Build history of the part. All positions in model axes, mm. Coordinates: 2 decimals unless noted, no trailing zeros. Loops run counter-clockwise (first coordinate to the right, second up) from the corner with the lowest first, then second, coordinate; pieces in that order, holes last.
Item 1: Cut at A-A (x = 17). List the corners of the cut face in (y, z), and give its area (3 significant figures).
Item 2: Mould opens along Y. For faces 1 (the face through (61.625, 0.33, 7.493)), 2 (the face through (111.122, -0.205, -0.427)), 3 (the face through (0, 0, 0)), 4 (the face through (123.36, -0.21, 0.18)) say: released by +Y, released by -Y, zero draft, split by the parting line, or undercut.
Item 3: Drill centre lines: line 1 along X through (y, z) = (-0.75, 0.25); line 2 along X through (y, z) = (-0.75, -0.5); line 3 along Z through (x, y) = (90, -0.25). Where is each one in solid material? Low to high.
Item 4: Flat gauge pins, fed straight in: pin 1 (6 mm diameter, centred on x = 62.5, z = -5, fed in from -Y); pin 2 (5 mm diameter, centred on x = 12.5, z = -4, fed in from +Y); pin 3 (8 mm diameter, centred on x = 43.5, y = 4, fed in from +Z); pin 4 (6 mm diameter, centred on x = 108.5, z = -4, fed in from +Y). Where does each tip first touch, or does it go through?
from build123d import *

# Parameters (mm, degrees)
SKETCH1_R                       = 7.5
BOSS_EXTRUDE1_DEPTH             = 125
F_3_32_0_09375_DIAMETER_HOLE1_D = 2.38125
F_2MM_DIAMETER_HOLE_D           = 2


with BuildPart() as part:
    # Sketch1 → Boss-Extrude1 (new body)
    with BuildSketch(Plane(origin=(0, 0, 0), x_dir=(0, 0, -1), z_dir=(1, 0, 0))):
        Circle(SKETCH1_R)
    extrude(amount=BOSS_EXTRUDE1_DEPTH)

    # 3/32 (0.09375) Diameter Hole1 (through all)
    with Locations(Plane(origin=(122.197095896, -2.4168895, -7.099904587), x_dir=(0, -0.946653944928, 0.322251933358), z_dir=(0, -0.322251933358, -0.946653944928))):
        with Locations((0, 0)):
            Hole(F_3_32_0_09375_DIAMETER_HOLE1_D / 2)

    # 2mm Diameter Hole (through all)
    with Locations(Plane(origin=(112.009618943, 7.312828958, -1.665092378), x_dir=(0, 0.222012317051, 0.975043861105), z_dir=(0, 0.975043861105, -0.222012317051))):
        with Locations((0, 0)):
            Hole(F_2MM_DIAMETER_HOLE_D / 2)


solid = part.part
Filled sheet:
1. outline: circle Ø15 at (0, 0)
1. area: 177 mm2
2. face 1: split by the parting line
2. face 2: undercut
2. face 3: zero draft
2. face 4: undercut
3. line 1: x = 0 to 111.01, 113.01 to 121.31, 123.09 to 125
3. line 2: x = 0 to 111.25, 112.77 to 121.14, 123.25 to 125
3. line 3: z = -7.5 to 7.5
4. pin 1: stops at y = -7.23
4. pin 2: stops at y = 7.35
4. pin 3: stops at z = 7.5
4. pin 4: stops at y = 7.43
